```python
from build123d import *

# Parameters (mm, degrees)
SKETCH1_R                       = 32.5
SKETCH1_R_2                     = 30.5
CYLINDER_BULK_EXTRUDE_DEPTH     = 90
TOP_START                       = -3
SKETCH2_R                       = 32.5
TOP_LID_DEPTH                   = 3
SKETCH3_R                       = 32.5
BOTTOM_LID_DEPTH                = 3
REAR_ACCESS_CUT_DEPTH           = 102.056914657
REAR_ACCESS_CUT_DEPTH_BACK      = 102.056914657
SKETCH5_W                       = 58.172158288
SKETCH5_H                       = 18
SKETCH8_W                       = 70
SKETCH8_H                       = 35
WEIGHT_RELIEF_PT1_DEPTH         = 102.056914657
CENTER_STIFFNESS_RIB_REACH      = 108.608
CENTER_STIFFNESS_RIB_END_RADIUS = 30.5
SKETCH6_W                       = 3
SKETCH6_H                       = 90
ALIGNMENT_SLOT_CUT_DEPTH        = 102.056914657
ALIGNMENT_SLOT_CUT_DEPTH_BACK   = 6
SKETCH4_W                       = 21
SKETCH4_H                       = 6
FILLET1_R                       = 1.5
SKETCH9_W                       = 20
SKETCH9_H                       = 5
ALIGNMENT_PEG_DEPTH             = 5
FILLET2_R                       = 1


with BuildPart() as part:
    # Sketch1 → CYLINDER BULK EXTRUDE (new body)
    with BuildSketch(Plane(origin=(0, 0, 0), x_dir=(1, 0, 0), z_dir=(0, 1, 0))):
        with Locations(Location((0, 0, 0), (0, 0, 90))):
            Circle(SKETCH1_R)
        with Locations(Location((0, 0, 0), (0, 0, 90))):
            Circle(SKETCH1_R_2, mode=Mode.SUBTRACT)
    extrude(amount=CYLINDER_BULK_EXTRUDE_DEPTH)

    # Sketch2 → TOP LID (add)
    with BuildSketch(Plane(origin=(0, 90, 0), x_dir=(1, 0, 0), z_dir=(0, 1, 0)).offset(TOP_START)):
        with Locations(Location((0, 0, 0), (0, 0, 90))):
            Circle(SKETCH2_R)
    extrude(amount=TOP_LID_DEPTH)

    # Sketch3 → BOTTOM LID (add)
    with BuildSketch(Plane.XZ):
        with Locations(Location((0, 0, 0), (0, 0, 270))):
            Circle(SKETCH3_R)
    extrude(amount=-BOTTOM_LID_DEPTH)

    # Sketch5 → REAR ACCESS CUT (cut, two sides: drawn at the far end of the back side and taken through both)
    with BuildSketch(Plane(origin=(0, 90, 0), x_dir=(1, 0, 0), z_dir=(0, 1, 0)).offset(-REAR_ACCESS_CUT_DEPTH_BACK)):
        with Locations((0, -23.5)):
            Rectangle(SKETCH5_W, SKETCH5_H)
    extrude(amount=REAR_ACCESS_CUT_DEPTH + REAR_ACCESS_CUT_DEPTH_BACK, mode=Mode.SUBTRACT)

    # Sketch8 → WEIGHT RELIEF PT1 (cut, symmetric)
    with BuildSketch(Plane(origin=(0, 0, 0), x_dir=(0, 1, 0), z_dir=(0.499999999999998, 0, -0.8660254037844398))):
        with Locations((40, 7.5)):
            Rectangle(SKETCH8_W, SKETCH8_H)
    weight_relief_pt1 = extrude(amount=WEIGHT_RELIEF_PT1_DEPTH, both=True, mode=Mode.SUBTRACT)

    # WEIGHT RELIEF PT2: WEIGHT RELIEF PT1 across plane
    add(weight_relief_pt1.mirror(Plane(origin=(0, 0, 0), x_dir=(0, 0, 1), z_dir=(1, 0, 0))), mode=Mode.SUBTRACT)

    # CENTER STIFFNESS RIB: up to this cylinder (the profile starts inside it)
    center_stiffness_rib_end = Plane(origin=(0, 45, 0), z_dir=(0, -1, 0)) * Cylinder(CENTER_STIFFNESS_RIB_END_RADIUS, 279.216, mode=Mode.PRIVATE)
    # Sketch6 → CENTER STIFFNESS RIB (add, up to the surface)
    with BuildSketch(Plane.XY.offset(14.5), mode=Mode.PRIVATE) as center_stiffness_rib_sk1:
        with Locations((0, 45)):
            Rectangle(SKETCH6_W, SKETCH6_H)
    center_stiffness_rib_tool1 = extrude(center_stiffness_rib_sk1.sketch, amount=-CENTER_STIFFNESS_RIB_REACH, mode=Mode.PRIVATE) & center_stiffness_rib_end
    add(center_stiffness_rib_tool1.solids().sort_by_distance((0, 45, 14.5))[0])

    # Sketch4 → ALIGNMENT SLOT CUT (cut, two sides: drawn at the far end of the back side and taken through both)
    with BuildSketch(Plane(origin=(0, 90, 0), x_dir=(1, 0, 0), z_dir=(0, 1, 0)).offset(-ALIGNMENT_SLOT_CUT_DEPTH_BACK)):
        with Locations((0, 20)):
            Rectangle(SKETCH4_W, SKETCH4_H)
    extrude(amount=ALIGNMENT_SLOT_CUT_DEPTH + ALIGNMENT_SLOT_CUT_DEPTH_BACK, mode=Mode.SUBTRACT)

    # Fillet1
    fillet1_edges = [part.edges().sort_by_distance(p)[0] for p in [
        (10.5, 90, -20),
        (-10.5, 90, -20),
        (0, 90, -17),
        (0, 90, -23),
    ]]
    fillet(fillet1_edges, radius=FILLET1_R)

    # Sketch9 → ALIGNMENT PEG (add)
    with BuildSketch(Plane.XZ):
        with Locations((0, -20)):
            Rectangle(SKETCH9_W, SKETCH9_H)
    extrude(amount=ALIGNMENT_PEG_DEPTH)

    # Fillet2
    fillet2_edges = [part.edges().sort_by_distance(p)[0] for p in [
        (-10, 0, -20),
        (0, 0, -22.5),
        (10, 0, -20),
        (0, 0, -17.5),
    ]]
    fillet(fillet2_edges, radius=FILLET2_R)


solid = part.part
```
Work out the finished part from the listing and answer in its coordinate system (mm). A direction names the side the tool comes from. Give positions to 0.01 mm unless a question says otherwise; leave off trailing zeros. Order: outer loops, then holes, each group sorted by start corner. A loop starts at its lowest first (then second) coordinate and runs counter-clockwise, first axis right, second up. Notation, with made-up numbers: M 82.25,-31.5 L 100.25,-31.5 A18 cw 100.25,-16.5 Z; hole C 55.25,65.25 d5. An arc over 180 degrees is marked long. Return JSON: item names as keys, results as strings.
1) Section D-D, the plane x = 24 is taken. Write down the section's boundary in (y, z), plus the area to 3 significant figures.
Resolved:
{"outline": "M 0,-21.91 L 5,-21.91 L 5,-18.82 L 3,-18.82 L 3,14.5 L 0,14.5 Z; M 75,-21.91 L 90,-21.91 L 90,14.5 L 87,14.5 L 87,-18.82 L 75,-18.82 Z", "area": "262 mm^2"}
2) For a pull along Z with two mould halves and no side action, classify faces 1 (the cylindrical face through (0.925, 44.37, -32.487)), 2 (the flat face through (0, 45, 14.5)), 3 (the flat face through (0, 87, -23)), 4 (the flat face through (10, -3, -20)) as +Z half, -Z half, draft (parallel to the pull), parting line (faces both ways), or undercut.
Resolved:
{"face 1": "parting line", "face 2": "+Z half", "face 3": "undercut", "face 4": "draft"}
3) Each of these flat-tipped pins is pushed along its axis until it touches: pin 1 (14.5 mm diameter, centred on x = 12.5, z = 2, fed in from -Y); pin 2 (1.2 mm diameter, centred on y = -2.5, z = -20, fed in from +X); pin 3 (10 mm diameter, centred on y = 45.5, z = -15, fed in from +X). Where does it stop, or does it pass through?
Resolved:
{"pin 1": "y = 0", "pin 2": "x = 10", "pin 3": "x = 1.5"}
4) Section B-B, the plane x = 0 is taken. Write down the section's boundary in (y, z).
Resolved:
{"outline": "M -5,-22.5 L -1,-22.5 A1 cw 0,-23.5 L 0,-32.5 L 90,-32.5 L 90,-24.5 A1.5 ccw 88.5,-23 L 84,-23 L 84,-17 L 88.5,-17 A1.5 ccw 90,-15.5 L 90,14.5 L 0,14.5 L 0,-16.5 A1 cw -1,-17.5 L -5,-17.5 Z"}
5) Straight lines are drawn through the part: line 1 along Y through (x, z) = (-13.5, 6); line 2 along X through (y, z) = (35.5, -2.5); line 3 along Y through (x, z) = (-9.5, -30). For each, find the intervals that lie inside material, in ascending order. Write a range as [from, to].
Resolved:
{"line 1": "[0, 3], [87, 90]", "line 2": "[-32.4, -30.4], [-1.5, 1.5], [30.4, 32.4]", "line 3": "[0, 5], [75, 90]"}
6) A tool of negligible diameter and unlimited length cuts with its end or side. For faces 5 (the flat face through (31.222, 39.51, -4.078)), 6 (the flat face through (0, 87, -17)), 7 (the cylindrical face through (30.46, 44.41, -1.55)), 8 (the flat face through (0, -3, -22.5)), from which of +Z, -Z, +X, -X, +Y, -Y can it reach the whole face along a straight path? Write none if from no direction.
Resolved:
{"face 5": "-Z", "face 6": "+Y", "face 7": "none", "face 8": "-Z, +X, -X, -Y"}
7) Section A-A, the plane z = 0 is taken. Write down the section's boundary in (x, y).
Resolved:
{"outline": "M -32.5,0 L 32.5,0 L 32.5,90 L -32.5,90 Z; hole M -30.5,3 L -1.5,3 L -1.5,87 L -30.5,87 Z; hole M 1.5,3 L 30.5,3 L 30.5,87 L 1.5,87 Z"}
8) Section C-C, the plane y = 49.5 is taken. Write down the section's boundary in (x, z).
Resolved:
{"outline": "M -32.03,-5.48 L -30.39,-2.63 A30.5 cw -26.83,14.5 L -29.09,14.5 A32.5 ccw Z; M -6.8,-31.78 A32.5 ccw 6.8,-31.78 L 5.75,-29.95 A30.5 cw 1.5,-30.46 L 1.5,14.5 L -1.5,14.5 L -1.5,-30.46 A30.5 cw -5.75,-29.95 Z; M 26.83,14.5 A30.5 cw 30.39,-2.63 L 32.03,-5.48 A32.5 ccw 29.09,14.5 Z"}
